Work out the finished part from the listing and answer in its coordinate system (mm). A direction names the side the tool comes from. Coordinates: 2 decimals unless noted, no trailing zeros. Order: outer loops, then holes, each group sorted by start corner. A loop starts at its lowest first (then second) coordinate and runs counter-clockwise, first axis right, second up. Notation, with made-up numbers: (71, 64.5) - (89, 64.5) arc R25 ccw to (89, 98.5) - close; hole circle Ø5 at (69.5, -27.5). An arc over 180 degrees is marked (long way). Answer as a JSON object with one key per item and string values. Group by question number.
1) Section D-D (y = -21) is taken. Give the vertices of the cut face in (x, z).
2) Section B-B (x = 36.5) is taken. Give the vertices of the cut face in (y, z).
3) A tool of negligible diameter and unlimited length cuts with its end or side. For faces 5 (the face through (27.65, -19.01, -44.03)), 6 (the face through (41.52, -38.71, -11.44)), from which of +Z, -Z, +X, -X, +Y, -Y can it reach the whole face along a straight path? Write none if from no direction.
4) The mould has two halves that part along X. Classify faces 1 (the face through (32.6, -9.13, -34.54)), 2 (the face through (15.83, -37.93, -10.19)), 3 (the face through (42.829, -16, -25)), 4 (the face through (-8.16, -39.01, -28.07)): released by +X, released by -X, zero draft, split by the parting line, or undercut.
5) Find the intervals of material crossed by line 1 along X through (y, z) = (-27, -40); line 2 along Y through (x, z) = (20.5, -42); line 3 along X through (y, z) = (-2.5, -37), in increasing order.
6) Section A-A (y = -26.5) is taken. Give the vertices of the cut face in (x, z), plus the area to 3 significant figures.
7) Section C-C (y = -16.5) is taken. Give the vertices of the cut face in (x, z), plus the area to 3 significant figures.
8) Each of these flat-tipped pins is pushed along its axis until it touches: P1, Ø3, axis at y = -25.5, z = -38, coming from the +X side; P2, Ø6, axis at x = 27.5, z = -40, coming from the -Y side; P3, Ø13, axis at x = 33, y = -32.5, coming from the -Z side. Where does it stop, or does it pass through?
from build123d import *

# Parameters (mm, degrees)
F0_W         = 52
F0_H         = 35
F1_DEPTH     = 40
F2_W         = 30
F2_H         = 18
F3_DEPTH     = 20
F4_R         = 5
F5_DEPTH     = 20.001
F6_SIZE      = 1.99999
F7_T1_DEPTH  = 40.1421556237
F7_T3_DEPTH  = 42.1421456237
F7_T5_DEPTH  = 46.00002
F7_T7_DEPTH  = 12.8284129826
F7_T9_DEPTH  = 54.1421456237
F7_T11_DEPTH = 58.00002
F7_T13_DEPTH = 52.1421556237


# Not quite as in the source:
# - a fillet or chamfer that OpenCascade refuses, or shapes differently, is made with other operations: its cross-section is extruded or revolved along the edge and cut away or added
# - a fillet or chamfer is up to 0.001 mm smaller than in the source, because OpenCascade refuses the exact size


with BuildPart() as f1:
    # F0 (on Front) → F1 (new body)
    with BuildSketch(Plane.XZ):
        with Locations((16.8289473057, -27.5394749641)):
            Rectangle(F0_W, F0_H)
    extrude(amount=F1_DEPTH)

    # F2 (on face) → F3 (cut)
    with BuildSketch(Plane.XZ.offset(40)):
        with Locations((27.8289473057, -36.0394749641)):
            Rectangle(F2_W, F2_H)
    extrude(amount=-F3_DEPTH, mode=Mode.SUBTRACT)

    # F4 (on face) → F5 (cut, through all)
    with BuildSketch(Plane.XZ.offset(20)):
        with Locations((27.8289473057, -36.0394749641)):
            Circle(F4_R)
    extrude(amount=-F5_DEPTH, mode=Mode.SUBTRACT)

    # F6 (size 2 in the source; OpenCascade refuses exactly that, so slightly less here)
    f6_edges = [f1.edges().sort_by_distance(p)[0] for p in [
        (-9.171053, -40, -27.539475),
        (16.828947, -40, -10.039475),
        (42.828947, -40, -18.539475),
        (27.828947, -40, -27.039475),
        (12.828947, -40, -36.039475),
        (1.828947, -40, -45.039475),
        (-9.171053, 0, -27.539475),
        (27.828947, -20, -45.039475),
        (12.828947, -20, -36.039475),
        (42.828947, -20, -36.039475),
        (27.828947, -20, -27.039475),
        (22.828947, -20, -36.039475),
        (42.828947, 0, -27.539475),
        (42.828947, -20, -10.039475),
        (42.828947, -30, -27.039475),
        (42.828947, -10, -45.039475),
        (12.828947, -30, -45.039475),
    ]]
    chamfer(f6_edges, length=F6_SIZE)

    # F7: fillet of radius 2 on 7 edges, made by hand

    # F7_s2 → F7_t1 (cut)
    with BuildSketch(Plane.XZ.offset(-0.0710778119)):
        with BuildLine():
            ThreePointArc((42.8289473057, -12.8678920889), (42.6767063707, -12.1025252242), (42.2431608681, -11.4536785265))
            Line((42.2431608681, -11.4536785265), (42.8289473057, -12.0394649641))
            Line((42.8289473057, -12.0394649641), (42.8289473057, -12.8678920889))
        make_face()
    extrude(amount=F7_T1_DEPTH, mode=Mode.SUBTRACT)

    # F7_s4 → F7_t3 (cut)
    with BuildSketch(Plane.XZ.offset(-2.0710678119)):
        with BuildLine():
            ThreePointArc((40.0005301809, -10.0394749641), (40.7658970457, -10.1917158991), (41.4147437433, -10.6252614018))
            Line((41.4147437433, -10.6252614018), (40.8289573057, -10.0394749641))
            Line((40.8289573057, -10.0394749641), (40.0005301809, -10.0394749641))
        make_face()
    extrude(amount=F7_T3_DEPTH, mode=Mode.SUBTRACT)

    # F7_s6 → F7_t5 (cut)
    with BuildSketch(Plane.XZ.offset(-3.00001)):
        with BuildLine():
            ThreePointArc((-9.1710526943, -12.0394749641), (-8.5852662567, -10.6252614018), (-7.1710526943, -10.0394749641))
            Line((-7.1710526943, -10.0394749641), (-9.1710526943, -10.0394749641))
            Line((-9.1710526943, -10.0394749641), (-9.1710526943, -12.0394749641))
        make_face()
    extrude(amount=F7_T5_DEPTH, mode=Mode.SUBTRACT)

    # F7_s8 → F7_t7 (cut)
    with BuildSketch(Plane(origin=(-0.0499974412, -0.0499974412, 0), x_dir=(0, 0, 1), z_dir=(-0.7071067812, -0.7071067812, 0))):
        with BuildLine():
            ThreePointArc((-12.0394749641, 5.0707070595), (-10.6252614018, 4.4849206218), (-10.0394749641, 3.0707070595))
            Line((-10.0394749641, 3.0707070595), (-10.0394749641, 5.0707070595))
            Line((-10.0394749641, 5.0707070595), (-12.0394749641, 5.0707070595))
        make_face()
    extrude(amount=F7_T7_DEPTH, mode=Mode.SUBTRACT)

    # F7_s10 → F7_t9 (cut)
    with BuildSketch(Plane.YZ.offset(-11.2421205062)):
        with BuildLine():
            ThreePointArc((-37.1715828753, -10.0394749641), (-37.93694974, -10.1917158991), (-38.5857964376, -10.6252614018))
            Line((-38.5857964376, -10.6252614018), (-38.00001, -10.0394749641))
            Line((-38.00001, -10.0394749641), (-37.1715828753, -10.0394749641))
        make_face()
    extrude(amount=F7_T9_DEPTH, mode=Mode.SUBTRACT)

    # F7_s12 → F7_t11 (cut)
    with BuildSketch(Plane.YZ.offset(-12.1710626943)):
        with BuildLine():
            ThreePointArc((0, -12.0394749641), (-0.5857864376, -10.6252614018), (-2, -10.0394749641))
            Line((-2, -10.0394749641), (0, -10.0394749641))
            Line((0, -10.0394749641), (0, -12.0394749641))
        make_face()
    extrude(amount=F7_T11_DEPTH, mode=Mode.SUBTRACT)

    # F7_s14 → F7_t13 (cut)
    with BuildSketch(Plane.YZ.offset(-9.2421305062)):
        with BuildLine():
            ThreePointArc((-40, -12.8678920889), (-39.847759065, -12.1025252242), (-39.4142135624, -11.4536785265))
            Line((-39.4142135624, -11.4536785265), (-40, -12.0394649641))
            Line((-40, -12.0394649641), (-40, -12.8678920889))
        make_face()
    extrude(amount=F7_T13_DEPTH, mode=Mode.SUBTRACT)


solid = f1.part
Report:
{
 "1": {"outline": "(-9.17, -45.04) - (11.83, -45.04) - (13.83, -43.04) - (13.83, -28.04) - (40.83, -28.04) - (42.83, -26.04) - (42.83, -12.87) arc R2 ccw to (42.24, -11.45) - (41.41, -10.63) arc R2 ccw to (40, -10.04) - (-7.17, -10.04) arc R2 ccw to (-9.17, -12.04) - close"},
 "2": {"outline": "(-40, -25.04) - (-38, -27.04) - (-22, -27.04) - (-20, -29.04) - (-20, -43.04) - (-18, -45.04) - (0, -45.04) - (0, -12.04) arc R2 ccw to (-2, -10.04) - (-37.17, -10.04) arc R2 ccw to (-38.59, -10.63) - (-39.41, -11.45) arc R2 ccw to (-40, -12.87) - close"},
 "3": {"face 5": "-Z, +X, -Y", "face 6": "+Z, +X, -Y"},
 "4": {"face 1": "undercut", "face 2": "zero draft", "face 3": "released by +X", "face 4": "released by -X"},
 "5": {"line 1": "x = -9.17 to 12.83", "line 2": "y = -20 to 0", "line 3": "x = -9.17 to 22.92, 32.74 to 42.83"},
 "6": {"outline": "(-9.17, -45.04) - (10.83, -45.04) - (12.83, -43.04) - (12.83, -27.04) - (40.83, -27.04) - (42.83, -25.04) - (42.83, -12.87) arc R2 ccw to (42.24, -11.45) - (41.41, -10.63) arc R2 ccw to (40, -10.04) - (-7.17, -10.04) arc R2 ccw to (-9.17, -12.04) - close", "area": "1,270 mm²"},
 "7": {"outline": "(-9.17, -45.04) - (40.83, -45.04) - (42.83, -43.04) - (42.83, -12.87) arc R2 ccw to (42.24, -11.45) - (41.41, -10.63) arc R2 ccw to (40, -10.04) - (-7.17, -10.04) arc R2 ccw to (-9.17, -12.04) - close; hole circle Ø10 at (27.83, -36.04)", "area": "1,740 mm²"},
 "8": {"P1": "stops at x = 12.83", "P2": "stops at y = -19.97", "P3": "stops at z = -27.04"}
}
